Autodesk Inventor part; units mm, degrees
ref_plane "YZ Plane" through (0, 0, 0) normal (1, 0, 0) x (0, 1, 0)
ref_plane "XZ Plane" through (0, 0, 0) normal (0, 1, 0) x (-1, 0, 0)
ref_plane "XY Plane" through (0, 0, 0) normal (0, 0, 1) x (1, 0, 0)
sketch "Sketch1" plane through (0, 0, 0) normal (0, 0, 1) x (1, 0, 0)
  line L0 (-22, -17) -> (22, -17)
  line L1 (22, -17) -> (22, 17)
  line L2 (22, 17) -> (-22, 17)
  line L3 (-22, 17) -> (-22, -17)
  line L4 (-22, -17) -> (22, 17) construction
  line L5 (22, -17) -> (-22, 17) construction
  point P0 (0, 0)
  dimension "d0" = 44
  dimension "d1" = 34
extrude "Extrusion1" add sketch "Sketch1" along normal blind 3
chamfer "Chamfer1" distance 5 angle 45 4 edges at (22, 17, 1.5) (-22, 17, 1.5) (22, -17, 1.5) (-22, -17, 1.5)
sketch "Sketch2" plane through (0, 0, 3) normal (0, 0, 1) x (1, 0, 0)
  line L0 (-13.5, -15.5) -> (13.5, -15.5)
  line L1 (13.5, -15.5) -> (13.5, 15.5)
  line L2 (13.5, 15.5) -> (-13.5, 15.5)
  line L3 (-13.5, 15.5) -> (-13.5, -15.5)
  line L4 (-13.5, -15.5) -> (13.5, 15.5) construction
  line L5 (13.5, -15.5) -> (-13.5, 15.5) construction
  point P0 (0, 0)
  dimension "d7" = 27
  dimension "d8" = 31
extrude "Extrusion2" add sketch "Sketch2" along normal blind 16
fillet "Fillet1" radius 3 4 edges at (13.5, -15.5, 11) (13.5, 15.5, 11) (-13.5, 15.5, 11) (-13.5, -15.5, 11)
sketch "Sketch3" plane through (0, 0, 0) normal (0, 0, -1) x (-1, 0, 0)
  line L0 (-18, 0) -> (18, 0) construction
  point P0 (0, 0)
  point P1 (0, 0)
  dimension "d12" = 36
hole "Hole1" at (18, 0, 0) at (-18, 0, 0) direction (0, 0, 1) diameter 3.4 depth 8 tip angle 118 countersink diameter 6.3 countersink angle 90
sketch "Sketch4" plane through (0, 0, 19) normal (0, 0, 1) x (1, 0, 0)
  line L0 (-3.15, 11) -> (3.15, 11)
  line L1 (3.15, 11) -> (3.15, 10)
  line L2 (3.15, 10) -> (-3.15, 10)
  line L3 (-3.15, 10) -> (-3.15, 11)
  line L4 (-3.15, 11) -> (3.15, 10) construction
  line L5 (3.15, 11) -> (-3.15, 10) construction
  line L6 (5.5, -3.15) -> (6.5, -3.15)
  line L7 (6.5, -3.15) -> (6.5, 3.15)
  line L8 (6.5, 3.15) -> (5.5, 3.15)
  line L9 (5.5, 3.15) -> (5.5, -3.15)
  line L10 (5.5, -3.15) -> (6.5, 3.15) construction
  line L11 (6.5, -3.15) -> (5.5, 3.15) construction
  line L12 (-9.15, -11) -> (-2.85, -11)
  line L13 (-2.85, -11) -> (-2.85, -10)
  line L14 (-2.85, -10) -> (-9.15, -10)
  line L15 (-9.15, -10) -> (-9.15, -11)
  line L16 (-9.15, -11) -> (-2.85, -10) construction
  line L17 (-2.85, -11) -> (-9.15, -10) construction
  point P0 (0, 0)
  point P1 (0, 10.5)
  point P2 (6, 0)
  point P3 (-6, -10.5)
  point P4 (0, 10.5)
  point P5 (6, 0)
  dimension "d20" = 6.3
  dimension "d21" = 1
  dimension "d22" = 1
  dimension "d23" = 6.3
  dimension "d24" = 6.3
  dimension "d25" = 1
  dimension "d26" = 10
  dimension "d27" = 6
  dimension "d28" = 10
  dimension "d29" = 6
extrude "Extrusion3" add sketch "Sketch4" along normal blind 10
sketch "Sketch5" plane through (0, 0, 0) normal (0, 0, -1) x (-1, 0, 0)
  line L0 (-10, -7.5) -> (10, -7.5)
  line L1 (10, -7.5) -> (10, 7.5)
  line L2 (10, 7.5) -> (-10, 7.5)
  line L3 (-10, 7.5) -> (-10, -7.5)
  line L4 (-10, -7.5) -> (10, 7.5) construction
  line L5 (10, -7.5) -> (-10, 7.5) construction
  point P0 (0, 0)
  dimension "d32" = 20
  dimension "d33" = 15
extrude "Extrusion4" cut sketch "Sketch5" against normal blind 10
fillet "Fillet2" radius 3 2 edges at (-10, -7.5, 5) (10, -7.5, 5)
chamfer "Chamfer2" distance 5 angle 45 2 edges at (-10, 7.5, 5) (10, 7.5, 5)
fillet "Fillet3" radius 3 4 edges at (10, 2.5, 5) (5, 7.5, 5) (-5, 7.5, 5) (-10, 2.5, 5)
sketch "Sketch6" plane through (0, 0, 10) normal (0, 0, -1) x (-1, 0, 0)
  line L0 (-1, 2) -> (1, 2)
  line L1 (1, 2) -> (1, 5.5)
  line L2 (1, 5.5) -> (-1, 5.5)
  line L3 (-1, 5.5) -> (-1, 2)
  line L4 (-6, -5.5) -> (-4, -5.5)
  line L5 (-4, -5.5) -> (-4, -2)
  line L6 (-4, -2) -> (-6, -2)
  line L7 (-6, -2) -> (-6, -5.5)
  line L8 (4, -5.5) -> (6, -5.5)
  line L9 (6, -5.5) -> (6, -2)
  line L10 (6, -2) -> (4, -2)
  line L11 (4, -2) -> (4, -5.5)
  line L12 (-4, -2) -> (4, -2) construction
  point P0 (0, 0)
  point P1 (0, 2)
  point P2 (0, -2)
  dimension "d41" = 2
  dimension "d42" = 2
  dimension "d43" = 2
  dimension "d44" = 3.5
  dimension "d45" = 3.5
  dimension "d46" = 2
  dimension "d47" = 2
  dimension "d48" = 8
extrude "Extrusion5" add sketch "Sketch6" along normal blind 8
chamfer "Chamfer3" distance 0.5 angle 45 12 edges at (5, -2, 2) (6, -3.75, 2) (4, -3.75, 2) (5, -5.5, 2) (0, 2, 2) (1, 3.75, 2) (0, 5.5, 2) (-1, 3.75, 2) (-4, -3.75, 2) (-5, -2, 2) (-6, -3.75, 2) (-5, -5.5, 2)
properties part number "Netzstecker"
The listing builds one solid part. Answer for the finished solid, in the listing's coordinates (mm). A direction names the side the tool comes from. Give positions to 0.01 mm unless a question says otherwise; leave off trailing zeros. Order: outer loops, then holes, each group sorted by start corner. A loop starts at its lowest first (then second) coordinate and runs counter-clockwise, first axis right, second up. Notation, with made-up numbers: (-9.5, 7.25) - (18.5, 7.25) arc R10 cw to (18.5, 12.25) - close; hole circle Ø9 at (64, -12). An arc over 180 degrees is marked (long way). Use one line per item in the form item = value.
1) Find section C-C on y = 0. Determine the outline of the cut face in (x, z).
Verdict:
outline = (-22, 0) - (-21.15, 0) - (-19.7, 1.45) - (-19.7, 3) - (-22, 3) - close; (-16.3, 1.45) - (-14.85, 0) - (-10, 0) - (-10, 10) - (10, 10) - (10, 0) - (14.85, 0) - (16.3, 1.45) - (16.3, 3) - (13.5, 3) - (13.5, 19) - (6.5, 19) - (6.5, 29) - (5.5, 29) - (5.5, 19) - (-13.5, 19) - (-13.5, 3) - (-16.3, 3) - close; (19.7, 1.45) - (21.15, 0) - (22, 0) - (22, 3) - (19.7, 3) - close
2) Find section B-B on z = 25.5. Determine the outline of the cut face in (x, y).
Verdict:
outline = (-9.15, -11) - (-2.85, -11) - (-2.85, -10) - (-9.15, -10) - close; (-3.15, 10) - (3.15, 10) - (3.15, 11) - (-3.15, 11) - close; (5.5, -3.15) - (6.5, -3.15) - (6.5, 3.15) - (5.5, 3.15) - close
3) Find section A-A on z = 8.75. Give the number of separate pieces and of enclosed holes in the cut face, and give its area (3 significant figures).
Verdict:
separate_pieces = 4
enclosed_holes = 1
area = 580 mm^2
4) Each of these flat-tipped pins is pushed along its axis until it touches: pin 1 (12 mm diameter, centred on y = -0.5, z = 24.5, fed in from -X); pin 2 (1.8 mm diameter, centred on y = -4, z = 4.5, fed in from +X); pin 3 (4 mm diameter, centred on x = -1.5, y = -7.5, fed in from +Z); pin 4 (2 mm diameter, centred on x = -18, y = 0, fed in from -Z). Where does it stop, or does it pass through?
Verdict:
pin_1 = -13.5
pin_2 = 13.5
pin_3 = 19
pin_4 = through
5) Find section D-D on x = 18. Determine the outline of the cut face in (y, z), and give its area (3 significant figures).
Verdict:
outline = (-16, 0) - (-3.15, 0) - (-1.7, 1.45) - (-1.7, 3) - (-16, 3) - close; (1.7, 1.45) - (3.15, 0) - (16, 0) - (16, 3) - (1.7, 3) - close
area = 83.7 mm^2
6) The mould has two halves that part along X. Classify faces 5 (the flat face through (-13.5, 0, 11)), 6 (the flat face through (-5, -5.5, 6)), 7 (the flat face through (6, -3.15, 24)): released by +X, released by -X, zero draft, split by the parting line, or undercut.
Verdict:
face_5 = released by -X
face_6 = undercut
face_7 = zero draft
7) For faces 1 (the flat face through (-6, -11, 24)), 2 (the flat face through (0, 8, 0)), 3 (the flat face through (7.5, 5, 4.9)), 4 (the cylindrical face through (12.64, 14.6, 11.11)), determine the directions among +Z, -Z, +X, -X, +Y, -Y from which every point of the face is accessible in a straight line to the end or side of a thin tool.
Verdict:
face_1 = +Z, +X, -X, -Y
face_2 = -Z, +X, -X, +Y, -Y
face_3 = -Z
face_4 = +Z, +X, +Y
8) Consider probe 1 along X at (y, z) = (0, 2.65); probe 2 along Z at (x, y) = (3, -1); probe 3 along Y at (x, z) = (18, 2.7). Determine where each line is inside the solid, lowest interval first. Write a range as [from, to].
Verdict:
probe_1 = [-22, -19.7], [-16.3, -10], [10, 16.3], [19.7, 22]
probe_2 = [10, 19]
probe_3 = [-16, -1.7], [1.7, 16]
